Study the drawing (mm; zero at the part's minimum x, y, z) and answer. Give positions to 0.01 mm unless a question says otherwise; leave off trailing zeros. Write each loop counter-clockwise with the first axis right and the second up, starting at its lowest first coordinate (ties: lowest second). Pieces come first, ordered by that corner, then holes. Notation, with made-up numbers: (-24.5, 38) - (7.5, 38) arc R26 ccw to (7.5, 72) - close; hole circle Ø3 at (88.5, 48.25). An arc over 180 degrees is marked (long way). Answer as CSV lines item,"result".
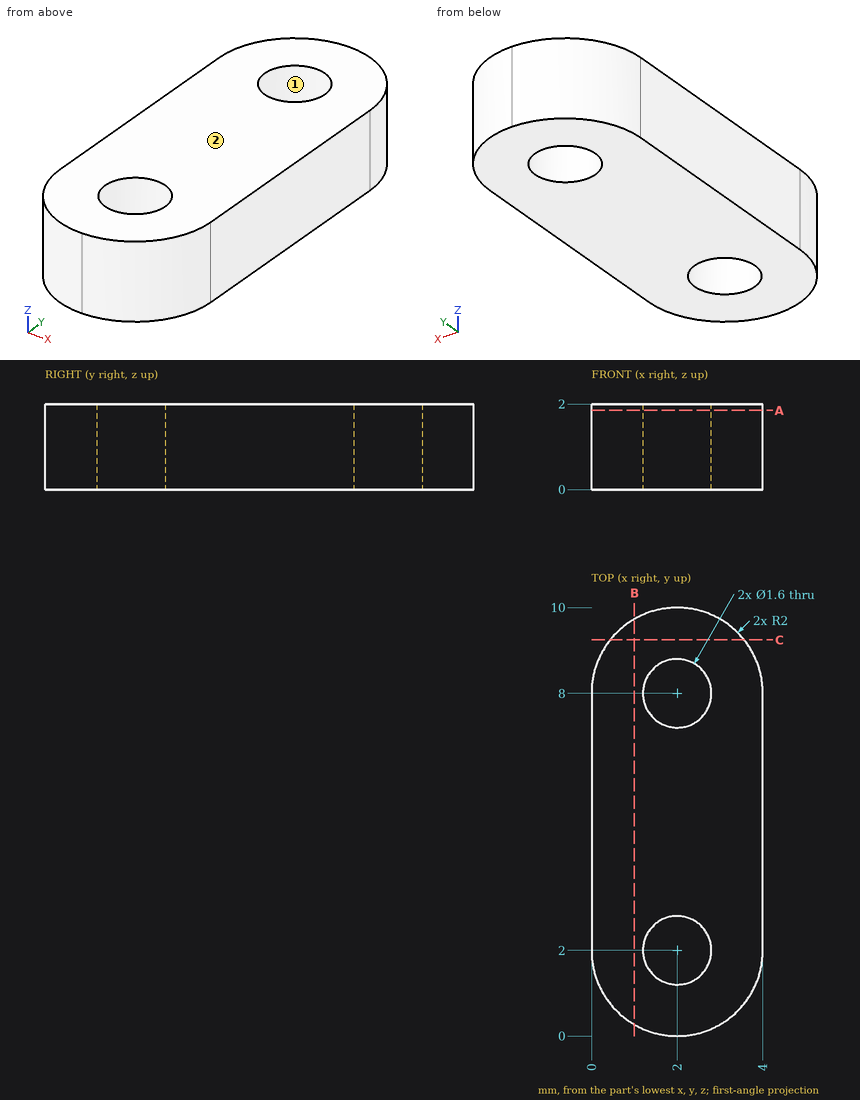
(1) Find the intervals of material crossed by L1, parallel to Y at x = 2, z = 0.45; L2, parallel to Y at x = 2.45, z = 1.4; L3, parallel to X at y = 2.25, z = 1.25, in increasing order.
Worked out:
L1,"y = 0 to 1.2, 2.8 to 7.2, 8.8 to 10"
L2,"y = 0.05 to 1.34, 2.66 to 7.34, 8.66 to 9.95"
L3,"x = 0 to 1.24, 2.76 to 4"
(2) A cutting plane is placed at B-B (x = 1). Write down the section's boundary in (y, z).
Worked out:
outline,"(0.27, 0) - (9.73, 0) - (9.73, 2) - (0.27, 2) - close"
(3) The mould has two halves that part along Y. Classify the marked faces 1 and 2: +Y half, -Y half, draft (parallel to the pull), parting line (faces both ways), or undercut.
Worked out:
face 1,"undercut"
face 2,"draft"
(4) This flat-tipped pin is pushed along its axis until it touches: P1, Ø1.3, axis at x = 2, y = 8, coming from the +Z side. Where does it stop, or does it pass through?
Worked out:
P1,"passes through"
(5) A cutting plane is placed at C-C (y = 9.25). Write down the section's boundary in (x, z), and give its area (4 significant figures).
Worked out:
outline,"(0.44, 0) - (3.56, 0) - (3.56, 2) - (0.44, 2) - close"
area,"6.245 mm^2"
(6) A cutting plane is placed at A-A (z = 1.85). Write down the section's boundary in (x, y).
Worked out:
outline,"(0, 2) arc R2 ccw to (4, 2) - (4, 8) arc R2 ccw to (0, 8) - close; hole circle Ø1.6 at (2, 2); hole circle Ø1.6 at (2, 8)"
